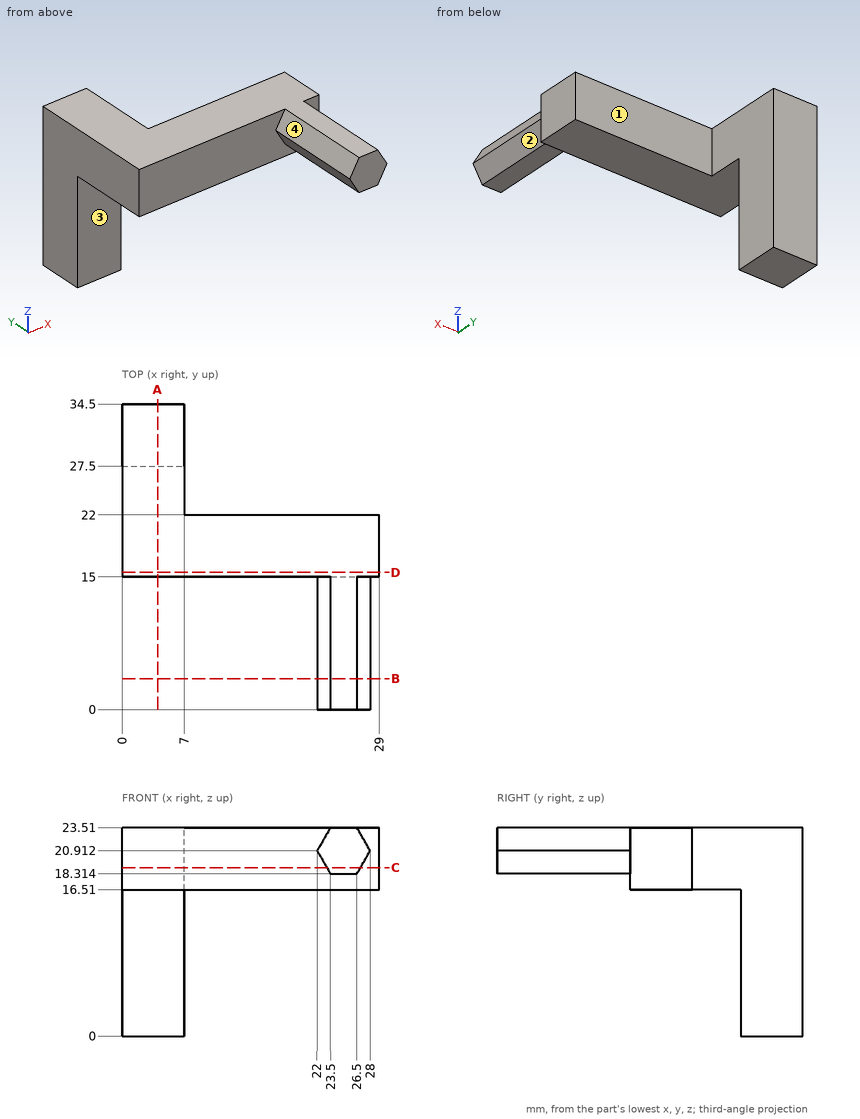
Design review of the part shown in the three views and the two pictorial views. Dimensions are in mm from the part's minimum x, y and z. A direction names the side the tool comes from. Coordinates: 2 decimals unless noted, no trailing zeros. Order: outer loops, then holes, each group sorted by start corner. A loop starts at its lowest first (then second) coordinate and runs counter-clockwise, first axis right, second up. Notation, with made-up numbers: (28, 56) -> (62, 56) arc R17 cw to (62, 69) -> close; hole circle Ø2 at (89, -10.75). An arc over 180 degrees is marked (long way). Use one line per item in the form item = value. Start each with the question number.
(1) Add section A-A on x = 4. State the section outline as (y, z) points, plus the area to 3 significant figures.
(2) Add section B-B on y = 3.5. State the section outline as (x, z) points, plus the area to 3 significant figures.
(3) For probe 1 along Y at (x, z) = (2.75, 2.25); probe 2 along X at (y, z) = (31.5, 16.25); probe 3 along Y at (x, z) = (17.25, 16.75), list the stretches that pass through material, from the lowest coordinate up.
(4) For the marked faces 1, 2, 3 and 4, list the 3-axis set-ups (+Z, -Z, +X, -X, +Y, -Y) from which the entire face can be reached by the end or side of a thin tool; tool diameter is ignored.
(5) Add section C-C on z = 19. State the section outline as (x, y) points.
(6) Add section D-D on y = 15.5. State the section outline as (x, z) points, plus the area to 3 significant figures.
(7) Insertion check: pin 1 (1.5 mm diameter, centred on y = 27, z = 19, fed in from +X); pin 2 (2 mm diameter, centred on x = 7.5, z = 11, fed in from +Y); pin 3 (6 mm diameter, centred on x = 20.5, y = 19.5, fed in from -Z); pin 4 (1.5 mm diameter, centred on y = 10, z = 19.5, fed in from +X). Each pin has a flat end and moves straight along its axis. Give the tip position at first contact, or say it passes through.
Answer block:
q1.outline = (15, 16.51) -> (27.5, 16.51) -> (27.5, 0) -> (34.5, 0) -> (34.5, 23.51) -> (15, 23.51) -> close
q1.area = 252 mm²
q2.outline = (22, 20.91) -> (23.5, 18.31) -> (26.5, 18.31) -> (28, 20.91) -> (26.5, 23.51) -> (23.5, 23.51) -> close
q2.area = 23.4 mm²
q3.probe_1 = 27.5 to 34.5
q3.probe_2 = 0 to 7
q3.probe_3 = 15 to 22
q4.face_1 = +Z, -Z, +X, +Y
q4.face_2 = -Z, +X, -Y
q4.face_3 = -Z, +X, -X, -Y
q4.face_4 = +Z, -X, -Y
q5.outline = (0, 15) -> (23.1, 15) -> (23.1, 0) -> (26.9, 0) -> (26.9, 15) -> (29, 15) -> (29, 22) -> (7, 22) -> (7, 34.5) -> (0, 34.5) -> close
q6.outline = (0, 16.51) -> (29, 16.51) -> (29, 23.51) -> (0, 23.51) -> close
q6.area = 203 mm²
q7.pin_1 = 7
q7.pin_2 = 34.5
q7.pin_3 = 16.51
q7.pin_4 = 27.62
